CAD build for the part. Positions are in the model's coordinates, mm. Face numbers are marked on the shaded views. A direction names the side the tool comes from. Round coordinates to 2 decimals unless told otherwise and drop trailing zeros. Order: outer loops, then holes, each group sorted by start corner. A loop starts at its lowest first (then second) coordinate and runs counter-clockwise, first axis right, second up. Notation, with made-up numbers: M 70.25,-33 L 118.25,-33 A17 cw 118.25,-10 Z; hole C 29,24 d1. An arc over 180 degrees is marked long. Answer as a JSON object with one key per item and string values.
Autodesk Inventor part; units mm, degrees
ref_plane "YZ Plane" through (0, 0, 0) normal (1, 0, 0) x (0, 1, 0)
ref_plane "XZ Plane" through (0, 0, 0) normal (0, 1, 0) x (-1, 0, 0)
ref_plane "XY Plane" through (0, 0, 0) normal (0, 0, 1) x (1, 0, 0)
sketch "Sketch1" plane through (0, 0, 0) normal (0, 0, 1) x (1, 0, 0)
  line L0 (22.5, 44) -> (22.5, 25.6111)
  line L1 (13.5, 44) -> (13.5, 29.9618)
  arc A0 (22.5, 18.6538) -> (13.5, 23.9242) centre (0, -9.4487) ccw
  arc A1 (34.7379, 0) -> (22.5, 18.6538) centre (0, -9.4487) ccw
  arc A2 (40.5729, 0) -> (22.5, 25.6111) centre (0, -9.4487) ccw
  line L2 (13.5, 29.9618) -> (13.5, 23.9242)
  line L3 (13.5, 44) -> (22.5, 44)
  line L4 (34.7379, 0) -> (40.5729, 0)
  line L5 (0, -20.1384) -> (0, 54.6897)
  point P0 (0, 0)
revolve "Revolution1" add sketch "Sketch1" angle 360 about axis through (0, -10, 0) along (0, 1, 0)
sketch "Sketch2" plane through (0, 44, 0) normal (0, 1, 0) x (1, 0, 0)
  line L0 (-7, -13.5) -> (-7, -36)
  line L1 (-7, -36) -> (7, -36)
  line L2 (7, -36) -> (7, -13.5)
  line L3 (7, -13.5) -> (7, -11.5434)
  circle A0 centre (0, 0) radius 13.5
  line L4 (-7, -13.5) -> (-7, -11.5434)
  line L5 (-7, 13.5) -> (-7, 36)
  line L6 (-7, 36) -> (7, 36)
  line L7 (7, 36) -> (7, 13.5)
  line L8 (-7, 13.5) -> (-7, 11.5434)
  line L9 (7, 13.5) -> (7, 11.5434)
  dimension "d12" = 14
  dimension "d13" = 22.5
  dimension "d16" = 14
  dimension "d17" = 22.5
extrude "Extrusion1" add sketch "Sketch2" against normal blind 7.5 contours L4 A0 L3 L2 L1 L0 | L8 L5 L6 L7 L9 A0
sketch "Sketch3" plane through (-7, 44, -36) normal (0, 1, 0) x (1, 0, 0)
  circle A0 centre (7, -66.0778) radius 2.8
  circle A1 centre (7.0706, -5.9222) radius 2.8
  line L0 (14, -14.6166) -> (14, 0)
  point P0 (7, -36)
  dimension "d20" = 5.6
  dimension "d21" = 5.6
extrude "Extrusion2" cut sketch "Sketch3" against normal blind 7.5
sketch "Sketch4" plane through (0, 0, 0) normal (0, -1, 0) x (1, 0, 0)
  circle A0 centre (0, 0) radius 40.5729
extrude "Extrusion3" add sketch "Sketch4" along normal blind 7
sketch "Sketch5" plane through (0, -7, 0) normal (0, -1, 0) x (1, 0, 0)
  arc A0 (16.1775, -12.0133) -> (16.301, -12.0133) centre (16.2392, -12.0133) ccw
  arc A1 (16.301, -12.0133) -> (16.1775, -12.0133) centre (16.2392, -12.0133) ccw
  arc A2 (23.9531, -12.0133) -> (24.0765, -12.0133) centre (24.0148, -12.0133) ccw
  arc A3 (24.0765, -12.0133) -> (23.9531, -12.0133) centre (24.0148, -12.0133) ccw
  arc A4 (24.0148, -12.0133) -> (16.2392, -12.0133) centre (20.127, -12.0133) ccw
  arc A5 (16.2392, -12.0133) -> (24.0148, -12.0133) centre (20.127, -12.0133) ccw
  arc A6 (19.3718, -10.1309) -> (11.5963, -10.1309) centre (15.484, -10.1309) ccw
  arc A7 (11.5963, -10.1309) -> (19.3718, -10.1309) centre (15.484, -10.1309) ccw
  arc A8 (19.3101, -10.1309) -> (19.4335, -10.1309) centre (19.3718, -10.1309) ccw
  arc A9 (19.4335, -10.1309) -> (19.3101, -10.1309) centre (19.3718, -10.1309) ccw
  arc A10 (12.4208, 8.2206) -> (12.5442, 8.2206) centre (12.4825, 8.2206) ccw
  arc A11 (12.5442, 8.2206) -> (12.4208, 8.2206) centre (12.4825, 8.2206) ccw
  arc A12 (20.1963, 8.2206) -> (20.3198, 8.2206) centre (20.2581, 8.2206) ccw
  arc A13 (20.3198, 8.2206) -> (20.1963, 8.2206) centre (20.2581, 8.2206) ccw
  arc A14 (16.3725, 11.3003) -> (16.496, 11.3003) centre (16.4342, 11.3003) ccw
  arc A15 (16.496, 11.3003) -> (16.3725, 11.3003) centre (16.4342, 11.3003) ccw
  arc A16 (20.2581, 8.2206) -> (12.4825, 8.2206) centre (16.3703, 8.2206) ccw
  arc A17 (12.4825, 8.2206) -> (20.2581, 8.2206) centre (16.3703, 8.2206) ccw
  arc A18 (24.1481, 11.3003) -> (24.2715, 11.3003) centre (24.2098, 11.3003) ccw
  arc A19 (24.2715, 11.3003) -> (24.1481, 11.3003) centre (24.2098, 11.3003) ccw
  arc A20 (24.2098, 11.3003) -> (16.4342, 11.3003) centre (20.322, 11.3003) ccw
  arc A21 (16.4342, 11.3003) -> (24.2098, 11.3003) centre (20.322, 11.3003) ccw
  arc A22 (-16.4271, -11.6758) -> (-16.3037, -11.6758) centre (-16.3654, -11.6758) ccw
  arc A23 (-16.3037, -11.6758) -> (-16.4271, -11.6758) centre (-16.3654, -11.6758) ccw
  arc A24 (-12.4137, -8.5961) -> (-20.1892, -8.5961) centre (-16.3014, -8.5961) ccw
  arc A25 (-20.1892, -8.5961) -> (-12.4137, -8.5961) centre (-16.3014, -8.5961) ccw
  arc A26 (-20.2509, -8.5961) -> (-20.1275, -8.5961) centre (-20.1892, -8.5961) ccw
  arc A27 (-20.1275, -8.5961) -> (-20.2509, -8.5961) centre (-20.1892, -8.5961) ccw
  arc A28 (-12.4754, -8.5961) -> (-12.3519, -8.5961) centre (-12.4137, -8.5961) ccw
  arc A29 (-12.3519, -8.5961) -> (-12.4754, -8.5961) centre (-12.4137, -8.5961) ccw
  arc A30 (3.7067, -23.2293) -> (-4.0688, -23.2293) centre (-0.181, -23.2293) ccw
  arc A31 (-4.0688, -23.2293) -> (3.7067, -23.2293) centre (-0.181, -23.2293) ccw
  arc A32 (3.0359, -18.5391) -> (-4.7397, -18.5391) centre (-0.8519, -18.5391) ccw
  arc A33 (-4.7397, -18.5391) -> (3.0359, -18.5391) centre (-0.8519, -18.5391) ccw
  arc A34 (-24.2027, -11.6758) -> (-24.0792, -11.6758) centre (-24.1409, -11.6758) ccw
  arc A35 (-24.0792, -11.6758) -> (-24.2027, -11.6758) centre (-24.1409, -11.6758) ccw
  arc A36 (-16.3654, -11.6758) -> (-24.1409, -11.6758) centre (-20.2532, -11.6758) ccw
  arc A37 (-24.1409, -11.6758) -> (-16.3654, -11.6758) centre (-20.2532, -11.6758) ccw
  arc A38 (-19.365, 9.7553) -> (-19.2416, 9.7553) centre (-19.3033, 9.7553) ccw
  arc A39 (-19.2416, 9.7553) -> (-19.365, 9.7553) centre (-19.3033, 9.7553) ccw
  arc A40 (-11.5277, 9.7553) -> (-19.3033, 9.7553) centre (-15.4155, 9.7553) ccw
  arc A41 (-19.3033, 9.7553) -> (-11.5277, 9.7553) centre (-15.4155, 9.7553) ccw
  arc A42 (-11.5894, 9.7553) -> (-11.466, 9.7553) centre (-11.5277, 9.7553) ccw
  arc A43 (-11.466, 9.7553) -> (-11.5894, 9.7553) centre (-11.5277, 9.7553) ccw
  arc A44 (-24.008, 11.6378) -> (-23.8845, 11.6378) centre (-23.9462, 11.6378) ccw
  arc A45 (-23.8845, 11.6378) -> (-24.008, 11.6378) centre (-23.9462, 11.6378) ccw
  arc A46 (-16.1707, 11.6378) -> (-23.9462, 11.6378) centre (-20.0585, 11.6378) ccw
  arc A47 (-23.9462, 11.6378) -> (-16.1707, 11.6378) centre (-20.0585, 11.6378) ccw
  arc A48 (-16.2324, 11.6378) -> (-16.109, 11.6378) centre (-16.1707, 11.6378) ccw
  arc A49 (-16.109, 11.6378) -> (-16.2324, 11.6378) centre (-16.1707, 11.6378) ccw
  arc A50 (-3.7405, 23.3979) -> (-3.617, 23.3979) centre (-3.6788, 23.3979) ccw
  arc A51 (-3.617, 23.3979) -> (-3.7405, 23.3979) centre (-3.6788, 23.3979) ccw
  arc A52 (4.0351, 23.3979) -> (4.1585, 23.3979) centre (4.0968, 23.3979) ccw
  arc A53 (4.1585, 23.3979) -> (4.0351, 23.3979) centre (4.0968, 23.3979) ccw
  arc A54 (4.0968, 23.3979) -> (-3.6788, 23.3979) centre (0.209, 23.3979) ccw
  arc A55 (-3.6788, 23.3979) -> (4.0968, 23.3979) centre (0.209, 23.3979) ccw
  arc A56 (-3.0289, 18.1638) -> (-2.9055, 18.1638) centre (-2.9672, 18.1638) ccw
  arc A57 (-2.9055, 18.1638) -> (-3.0289, 18.1638) centre (-2.9672, 18.1638) ccw
  arc A58 (4.7467, 18.1638) -> (4.8701, 18.1638) centre (4.8084, 18.1638) ccw
  arc A59 (4.8701, 18.1638) -> (4.7467, 18.1638) centre (4.8084, 18.1638) ccw
  arc A60 (4.8084, 18.1638) -> (-2.9672, 18.1638) centre (0.9206, 18.1638) ccw
  arc A61 (-2.9672, 18.1638) -> (4.8084, 18.1638) centre (0.9206, 18.1638) ccw
extrude "Extrusion4" cut sketch "Sketch5" against normal blind 1 contours A0 A5 A7 A6 A4 A1 | A5 A4 A1 A0 | A0 A1 A4 A6 A9 A8 A7 A5 | A7 A8 A9 A6 A4 A3 A2 A5 | A2 A3 A4 A5 | A8 A9 A6 A7 | A17 A16 A11 A10 | A10 A11 A16 A20 A15 A14 A21 A17 | A21 A14 A15 A20 A16 A13 A12 A17 | A17 A12 A13 A16 A20 A19 A18 A21 | A12 A13 A16 A17 | A21 A20 A15 A14 | A18 A19 A20 A21 | A23 A36 A37 A22 | A22 A37 A25 A26 A27 A24 A36 A23 | A22 A23 A36 A24 A29 A28 A25 A37 | A37 A34 A35 A36 A24 A27 A26 A25 | A25 A24 A27 A26 | A28 A29 A24 A25 | A37 A36 A35 A34 | A31 A30 A33 | A33 A30 | A30 A33 A32 | A38 A41 A47 A44 A45 A46 A40 A39 | A41 A40 A39 A38 | A38 A39 A40 A46 A49 A48 A47 A41 | A47 A48 A49 A46 A40 A43 A42 A41 | A42 A43 A40 A41 | A47 A46 A45 A44 | A48 A49 A46 A47 | A55 A54 A51 A50 | A50 A51 A54 A53 A52 A55 A60 | A60 A55 | A55 A60 A59 A58 A61 A56 A57 | A54 A55 A52 A53 | A57 A56 A61 A60 | A60 A61 A58 A59 picked at (16.2777, -12.003) picked at (23.9764, -12.0235) picked at (19.3334, -10.1207) picked at (12.5209, 8.2104) picked at (20.2196, 8.2103) picked at (16.4727, 11.3106) picked at (24.1714, 11.2901) picked at (-16.4038, -11.6656) picked at (-20.1508, -8.6063) picked at (-12.4521, -8.5859) picked at (-24.1025, -11.686) picked at (-19.2649, 9.7655) picked at (-11.5661, 9.7451) picked at (-23.9078, 11.6276) picked at (-16.2091, 11.648) picked at (-3.6403, 23.4082) picked at (4.0584, 23.4081) picked at (-2.9288, 18.1536) picked at (4.77, 18.174)
sketch "Sketch6" plane through (0, -7, 0) normal (0, -1, 0) x (1, 0, 0)
  point P0 (0, 0)
sketch "Sketch7" plane through (0, -7, 0) normal (0, -1, 0) x (1, 0, 0)
  point P0 (0, 0)
sketch "Sketch8" plane through (0, -7, 0) normal (0, -1, 0) x (1, 0, 0)
  point P0 (0, 0)
properties part number "Sensing gripper"
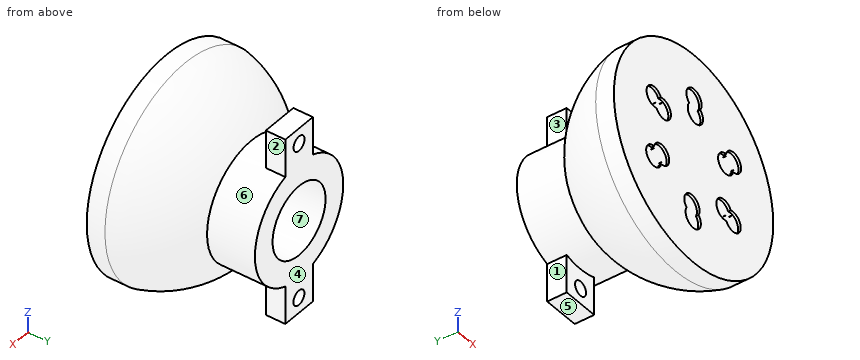
Item 1: Saw through at A-A on y = 30. List the corners of the cut face in (x, z), and give its area (3 significant figures).
Worked answers:
{"outline": "C 0,0 d45; hole C 0,0 d27", "area": "1,020 mm2"}
Item 2: Wall check: line 1 along Y through (x, z) = (-3.5, 32); line 2 along Z through (x, y) = (-2.5, 41); line 3 along X through (y, z) = (19.5, -15.5). Give the ranges that are in metal, low to high. Write a range as [from, to].
Worked answers:
{"line 1": "y = [-7, 0], [6.67, 16.99], [36.5, 44]", "line 2": "z = [-36, -31.19], [-28.97, -13.27], [13.27, 28.82], [31.34, 36]", "line 3": "x = [-25.64, -14.76], [14.76, 25.64]"}
Item 3: 3-axis set-ups, long thin cutter, end or side, ignore diameter. For the marked faces 1, 2 and 3: which of +Z, -Z, +X, -X, +Y, -Y reach the whole face in a straight line?
Worked answers:
{"face 1": "-Z, -X, +Y", "face 2": "+Z, +X, +Y", "face 3": "+Z, -X, +Y"}
Item 4: Saw through at B-B on x = 0. State how many separate pieces and enclosed holes the cut face has, and give its area (3 significant figures).
Worked answers:
{"separate pieces": "3", "enclosed holes": "0", "area": "1,380 mm2"}
Item 5: Two-plate mould, pull along Z, no slides. Class the marked faces 4, 5, 6 and 7: released by +Z, released by -Z, zero draft, split by the parting line, or undercut.
Worked answers:
{"face 4": "zero draft", "face 5": "released by -Z", "face 6": "split by the parting line", "face 7": "undercut"}
Item 6: Drop flat-ended pins along their axis: pin 1 Ø2 at (x, y) = (1.5, 10) entering from +Z; pin 2 Ø6 at (x, y) = (-1, 39.5) entering from +Z; pin 3 Ø4.5 at (x, z) = (-0.18, -23.23) entering from -Y. Give the stop position or say it passes through.
Worked answers:
{"pin 1": "stops at z = 37.32", "pin 2": "stops at z = 36", "pin 3": "stops at y = -6"}
